For this review, take the finished solid that the model builds, in its own axes (mm). Face numbers are marked on the shaded views. A direction names the side the tool comes from. Round coordinates to 2 decimals unless told otherwise and drop trailing zeros. Order: outer loops, then holes, each group sorted by start corner. A loop starts at its lowest first (then second) coordinate and runs counter-clockwise, first axis right, second up. Notation, with made-up numbers: (-1.5, 17) - (37.5, 17) arc R29 ccw to (37.5, 45) - close; hole circle Ø4 at (3, 71). An arc over 180 degrees is marked (long way). One line per item, written item: value.
```python
from build123d import *

# Parameters (mm, degrees)
SKETCH_R     = 1
SKETCH_W     = 23.3
SKETCH_H     = 12.8
PAD_DEPTH    = 4
SKETCH001_W  = 23.3
SKETCH001_H  = 6
PAD001_DEPTH = 13.5
SKETCH002_R  = 1.25
PAD002_DEPTH = 2
SKETCH003_R  = 1.4
POCKET_DEPTH = 11
FILLET_R     = 1
FILLET001_R  = 1


with BuildPart() as part:
    # Sketch → Pad (new body)
    with BuildSketch(Plane.XY):
        with BuildLine():
            Line((-17.65, 12.4), (14.65, 12.4))
            ThreePointArc((17.65, 9.4), (16.77132, 11.52132), (14.65, 12.4))
            ThreePointArc((26.84, 3.51), (22.883245, 7.450836), (17.65, 9.4))
            ThreePointArc((26.84, 3.51), (20.406481, 0.259943), (17.65, -6.4))
            ThreePointArc((14.65, -9.4), (16.77132, -8.52132), (17.65, -6.4))
            Line((14.65, -9.4), (-17.27, -9.4))
            ThreePointArc((-17.27, -9.4), (-43.226691, -0.259051), (-70.626477, -2.82))
            ThreePointArc((-72.67, 2.821276), (-74.470639, -1.021762), (-70.626477, -2.82))
            ThreePointArc((-17.65, 12.4), (-45.579054, 10.017677), (-72.67, 2.821276))
        make_face()
        with Locations((-14.15, 0)):
            Circle(SKETCH_R, mode=Mode.SUBTRACT)
        with Locations((14.15, 0)):
            Circle(SKETCH_R, mode=Mode.SUBTRACT)
        Rectangle(SKETCH_W, SKETCH_H, mode=Mode.SUBTRACT)
        with BuildLine():
            Line((17.65, 7.636176), (17.65, -0.84))
            ThreePointArc((23.88, 4.42), (20.301686, 2.338754), (17.65, -0.84))
            ThreePointArc((23.88, 4.42), (21.017458, 6.51712), (17.65, 7.636176))
        make_face(mode=Mode.SUBTRACT)
        with BuildLine():
            Line((-17.66615, -3.466269), (-17.66615, 4.388555))
            ThreePointArc((-17.66615, 4.388555), (-18.261027, 5.807615), (-19.69, 6.378267))
            ThreePointArc((-19.69, 6.378267), (-34.408413, 5.451456), (-48.98, 3.18))
            ThreePointArc((-19.59, -4.623545), (-33.83794, 0.961961), (-48.98, 3.18))
            ThreePointArc((-19.59, -4.623545), (-18.300889, -4.58882), (-17.66615, -3.466269))
        make_face(mode=Mode.SUBTRACT)
    extrude(amount=PAD_DEPTH)

    # Sketch001 (on Face24 of Pad) → Pad001 (join)
    with BuildSketch(Plane(origin=(0, 0, 0), x_dir=(1, 0, 0), z_dir=(0, 0, -1))):
        with Locations((0, -9.4)):
            Rectangle(SKETCH001_W, SKETCH001_H)
    extrude(amount=PAD001_DEPTH)

    # Sketch002 (on Face29 of Pad001) → Pad002 (join)
    with BuildSketch(Plane(origin=(0, 0, -13.5), x_dir=(1, 0, 0), z_dir=(0, 0, -1))):
        with Locations((-8.5, -9.4)):
            Circle(SKETCH002_R)
        with Locations((8.5, -9.4)):
            Circle(SKETCH002_R)
    extrude(amount=PAD002_DEPTH)

    # Sketch003 (on Face29 of Pad002) → Pocket (cut)
    with BuildSketch(Plane(origin=(0, 0, -13.5), x_dir=(1, 0, 0), z_dir=(0, 0, -1))):
        with Locations((0, -9.44)):
            Circle(SKETCH003_R)
    extrude(amount=-POCKET_DEPTH, mode=Mode.SUBTRACT)

    # Fillet
    fillet_edges = [part.edges().sort_by_distance(p)[0] for p in [
        (-11.65, 12.4, -6.75),
    ]]
    fillet(fillet_edges, radius=FILLET_R)

    # Fillet001
    fillet001_edges = [part.edges().sort_by_distance(p)[0] for p in [
        (11.65, 12.4, -6.75),
    ]]
    fillet(fillet001_edges, radius=FILLET001_R)


solid = part.part
```
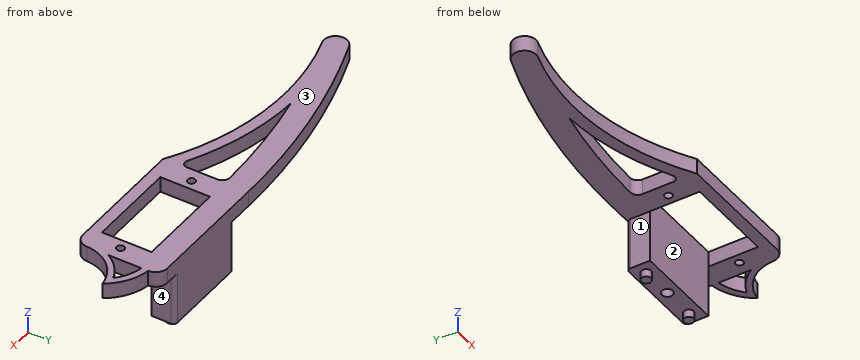
Item 1: Take a section at B-B (z = -11). Write out the cut boundary in (x, y), plus the area to 3 significant figures.
Returned:
outline: (-11.65, 6.4) - (11.65, 6.4) - (11.65, 11.4) arc R1 ccw to (10.65, 12.4) - (-10.65, 12.4) arc R1 ccw to (-11.65, 11.4) - close; hole circle Ø2.8 at (0, 9.44)
area: 133 mm^2
Item 2: Machinability: for the marked faces 1, 2, 3 and 4, which of the approach directions +Z, -Z, +X, -X, +Y, -Y give a long, thin tool a straight path to every point of the face, cutting with its end or side? Answer none if there is none.
Returned:
face 1: -Z, -X, +Y, -Y
face 2: +Z, -Z
face 3: +Z, +X, -X, +Y, -Y
face 4: -Z, +X, +Y, -Y
Item 3: Wall thickness on line 1 (X direction, y = 9.44, z = -5.5); line 2 (Y direction, x = 0, z = -6.75); line 3 (Y direction, x = 14.15, z = 0.85): over which ranges is each line inside the solid? List them lowest first.
Returned:
line 1: -11.65 to -1.4, 1.4 to 11.65
line 2: 6.4 to 8.04, 10.84 to 12.4
line 3: -9.4 to -1, 1 to 12.4
Item 4: Take a section at A-A (x = -4). Write out the cut boundary in (y, z).
Returned:
outline: (-9.4, 0) - (-6.4, 0) - (-6.4, 4) - (-9.4, 4) - close; (6.4, -13.5) - (12.4, -13.5) - (12.4, 4) - (6.4, 4) - close
Item 5: For P1, Ø1.2, axis at y = -1, z = 2, coming from the -X side; P2, Ø2.5, axis at y = 10, z = -6, coming from the +X side; P3, Ø1.8, axis at x = -1, y = 8.5, coming from the -Z side; P4, Ø4.5, axis at y = 2, z = 2.5, coming from the +X side, all flat-tipped, find the tip position at first contact; note any pin that passes through.
Returned:
P1: x = -74.62
P2: x = 11.65
P3: z = -13.5
P4: x = 26.84
Item 6: Take a section at C-C (x = -34). Write out the cut boundary in (y, z).
Returned:
outline: (-2.09, 0) - (1, 0) - (1, 4) - (-2.09, 4) - close; (5.5, 0) - (11.6, 0) - (11.6, 4) - (5.5, 4) - close
Item 7: Take a section at D-D (x = -71.65). Write out the cut boundary in (y, z), plus the area to 3 significant figures.
Returned:
outline: (-3, 0) - (3.19, 0) - (3.19, 4) - (-3, 4) - close
area: 24.7 mm^2
